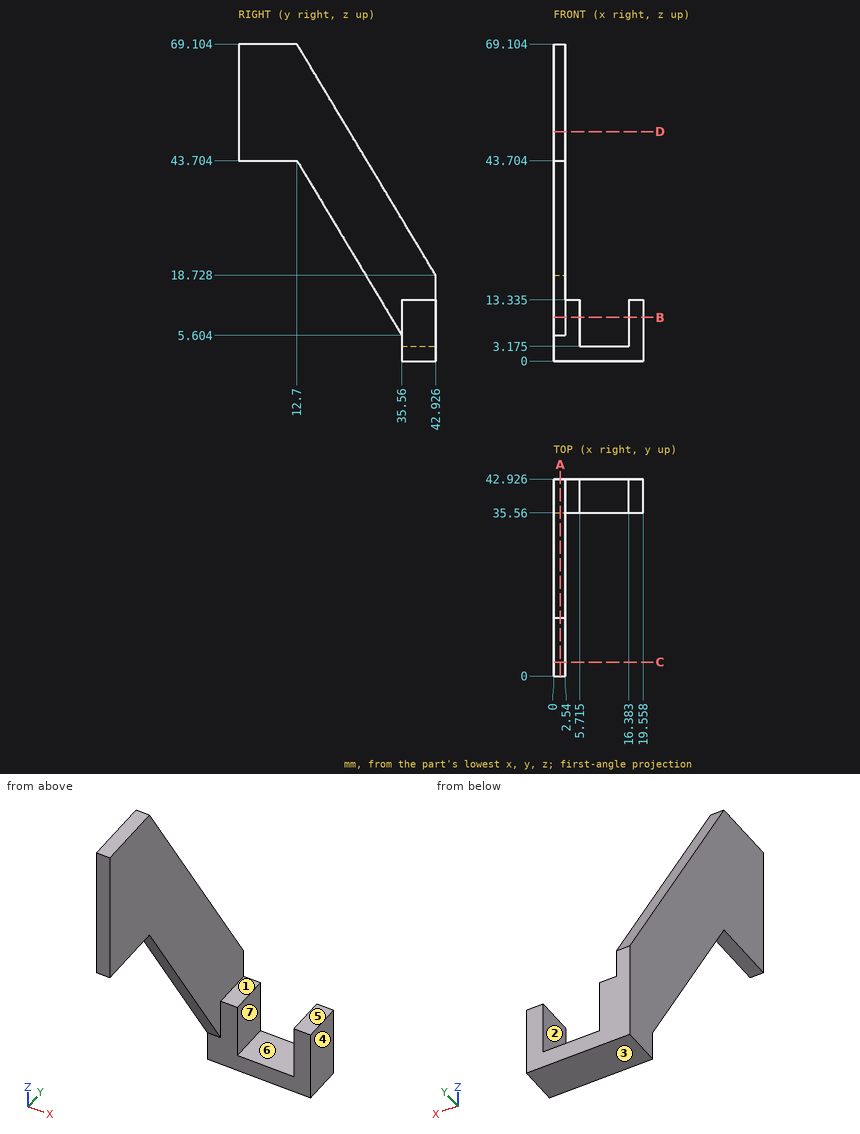
Here's the drawing with two shaded views (mm, measured from the low corner). I have some questions. A direction names the side the tool comes from. Round coordinates to 2 decimals unless told otherwise and drop trailing zeros. Order: outer loops, then holes, each group sorted by start corner. A loop starts at its lowest first (then second) coordinate and runs counter-clockwise, first axis right, second up. Notation, with made-up numbers: M -8,-9 L 10,-9 A22 cw 10,18 Z; hole C -27,69.25 d9. An arc over 180 degrees is marked long. Use CSV: the item, a comma, the result in double quotes.
1) On a 3-axis mill with a long thin cutter (end or side, diameter ignored), from which of +Z, -Z, +X, -X, +Y, -Y can I reach the whole of each face in a straight line? I mean the marked faces 1, 2 and 3. Say none if no direction works.
Taken from the geometry:
face 1,"+Z, +X, +Y, -Y"
face 2,"+Z, +Y, -Y"
face 3,"-Z, +X, -X, +Y, -Y"
2) If we mould it in two halves opening along X, with no side actions, what happens to the marked faces 4, 5, 6 and 7? For each: pulls with the +X half, pulls with the -X half, needs draft (parallel to the pull), parting line crosses it, or undercut.
Taken from the geometry:
face 4,"pulls with the +X half"
face 5,"needs draft"
face 6,"undercut"
face 7,"undercut"
3) I need wall thicknesses on line 1 along Y through (x, z) = (17.75, 4); line 2 along Z through (x, y) = (11.25, 36) (1 decimal); line 3 along X through (y, z) = (12.5, 52). Which ranges of each line are inside material? Lowest first, please. Write a range as [from, to].
Taken from the geometry:
line 1,"[35.56, 42.93]"
line 2,"[0, 3.2]"
line 3,"[0, 2.54]"
4) I'm going to push flat-ended pins straight in: P1, Ø1.5, axis at y = 4.5, z = 55.5, coming from the +X side; P2, Ø4, axis at x = 4, y = 7, coming from the +Z side; P3, Ø3, axis at x = 1, y = 7.5, coming from the -Z side; P4, Ø3.5, axis at x = 9.5, y = 40.5, coming from the +Z side (3 decimals). Where does each tip first touch, or does it pass through?
Taken from the geometry:
P1,"x = 2.54"
P2,"z = 69.1"
P3,"z = 43.7"
P4,"z = 3.175"
5) I want a section at D-D (z = 50). List the corners of the cut face in (x, y) for me.
Taken from the geometry:
outline,"M 0,0 L 2.54,0 L 2.54,24.16 L 0,24.16 Z"
6) I want a section at A-A (x = 1.5). List the corners of the cut face in (y, z) for me (1 decimal), then the cut area to 3 significant figures.
Taken from the geometry:
outline,"M 0,43.7 L 12.7,43.7 L 35.6,5.6 L 35.6,0 L 42.9,0 L 42.9,18.7 L 12.7,69.1 L 0,69.1 Z"
area,"1,090 mm^2"
7) I want a section at B-B (z = 9.5). List the corners of the cut face in (x, y) for me (1 decimal).
Taken from the geometry:
outline,"M 0,33.2 L 2.5,33.2 L 2.5,35.6 L 5.7,35.6 L 5.7,42.9 L 0,42.9 Z; M 16.4,35.6 L 19.6,35.6 L 19.6,42.9 L 16.4,42.9 Z"
8) I want a section at C-C (y = 3). List the corners of the cut face in (x, z) for me (1 decimal).
Taken from the geometry:
outline,"M 0,43.7 L 2.5,43.7 L 2.5,69.1 L 0,69.1 Z"
